Check sheet for the drawn part. Datum: minimum x, y, z corner. Units: mm. A direction names the side the tool comes from. Round coordinates to 2 decimals unless told otherwise and drop trailing zeros. Write each loop counter-clockwise with the first axis right and the second up, starting at its lowest first coordinate (ties: lowest second). Pieces come first, ordered by that corner, then holes. Notation, with made-up numbers: (-21.5, 55) - (16.5, 55) arc R37 cw to (16.5, 91) - close; hole circle Ø4 at (15.5, -8.5). An arc over 180 degrees is marked (long way). Answer as a JSON object with one key per item and string values. Group by question number.
1) Go/stop test with flat-tipped pins: pin 1 Ø8 at (y, z) = (38, 6.5) entering from +X; pin 2 Ø3 at (x, z) = (16.5, 13) entering from -Y; pin 3 Ø1 at (y, z) = (16.5, 5.5) entering from +X. Record where each tip stops, or that it passes through.
2) Thickness scan on line 1 (Z direction, x = 34.5, y = 47); line 2 (Y direction, x = 23.5, z = 1.75); line 3 (Y direction, x = 22, z = 21.25). Record the ranges inside material, lowest first.
3) Section check C-C (z = 2.75). Enter the section's corners in (x, y).
4) Section check D-D (z = 24.5). Enter the section's corners in (x, y).
5) Section check A-A (y = 30). Enter the section's corners in (x, z), then the cut area to 3 significant figures.
6) Set-up check for the marked faces 1 and 2: record each of +Z, -Z, +X, -X, +Y, -Y from which the full face is reachable in a straight line by a thin tool's end or side.
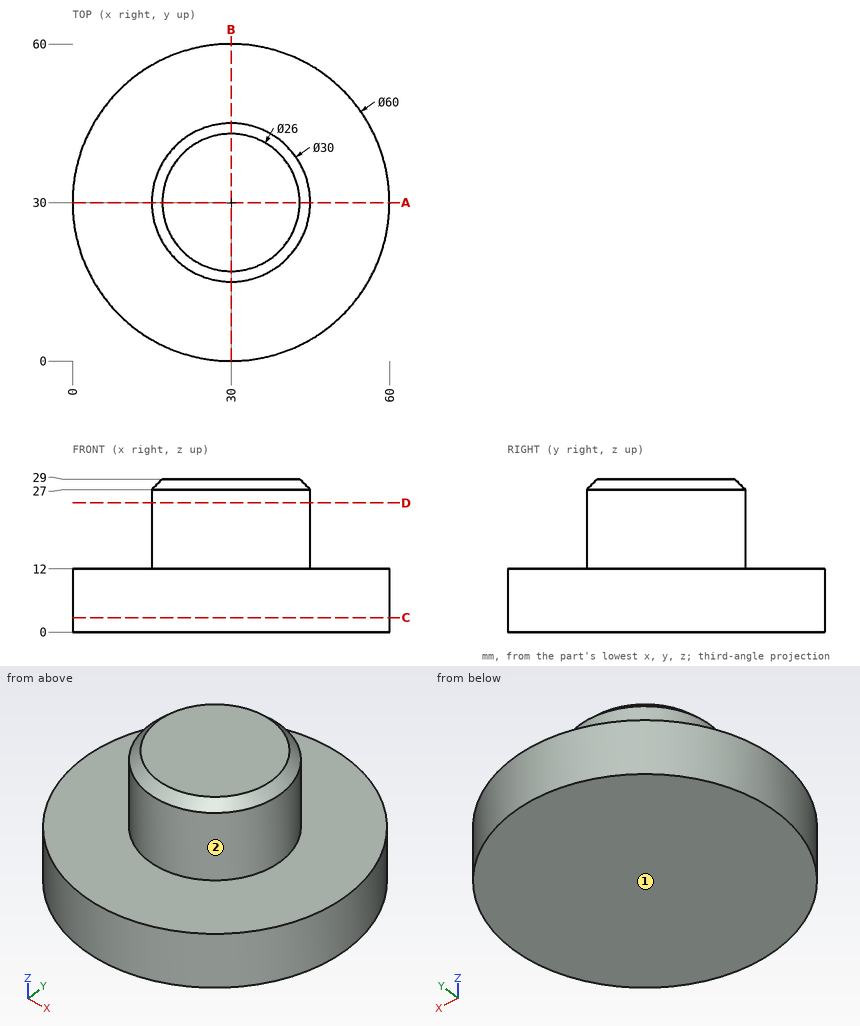
Returned:
{
 "1": {"pin 1": "x = 59.73", "pin 2": "y = 2.67", "pin 3": "x = 57.04"},
 "2": {"line 1": "0 to 12", "line 2": "0.71 to 59.29", "line 3": "17.31 to 42.69"},
 "3": {"outline": "circle Ø60 at (30, 30)"},
 "4": {"outline": "circle Ø30 at (30, 30)"},
 "5": {"outline": "(0, 0) - (60, 0) - (60, 12) - (45, 12) - (45, 27) - (43, 29) - (17, 29) - (15, 27) - (15, 12) - (0, 12) - close", "area": "1,230 mm2"},
 "6": {"face 1": "-Z, +X, -X, +Y, -Y", "face 2": "+Z"}
}
